CAD build for the part. Positions are in the model's coordinates, mm. A direction names the side the tool comes from. Coordinates: 2 decimals unless noted, no trailing zeros. Write each loop counter-clockwise with the first axis right and the second up, starting at its lowest first coordinate (ties: lowest second). Pieces come first, ordered by that corner, then holes. Notation, with made-up numbers: (14, -8) - (61, -8) arc R25 cw to (61, 20) - close; hole circle Ø5 at (12.5, 4.25). An arc over 180 degrees is marked (long way). One line per question, with ' | ' between items. Start each with the question number.
1. Two-plate mould, pull along X, no slides. Class faces 1 (the cylindrical face through (25.367, 8.972, -104.749)), 2 (the flat face through (-27, 7, -22)), 3 (the cylindrical face through (12.315, 5.423, -103.107)): +X half, -X half, draft (parallel to the pull), parting line (faces both ways), or undercut.
2. Which spindle directions (+Z, -Z, +X, -X, +Y, -Y) get a long thin tool onto all of the face, cutting with end or side? Do faces 4 (the cylindrical face through (-95.4, 2, -27.4)), 5 (the cylindrical face through (101.7, 2, -60.4)), 6 (the flat face through (1, 11, -63)), 7 (the cylindrical face through (-101.7, 2, -60.4)). Say none if no direction does.
3. Band-saw the part on A-A, the plane x = 65.5. Write the cut outline in (y, z), then the cut area to 3 significant figures.
4. Band-saw the part on B-B, the plane y = 4. Give the number of separate pieces and of enclosed holes in the cut face, then the cut area to 3 significant figures.
5. Flat gauge pins, fed straight in: P1, Ø1.5, axis at y = 2, z = -105.5, coming from the -X side; P2, Ø3, axis at x = -9.5, y = 15, coming from the -Z side. Where does each tip first touch, or does it go through?
6. Probe line 1 (X direction, y = 16, z = -30); line 2 (X direction, y = 16.75, z = -64); line 3 (X direction, y = 14.5, z = -64). List the from-to ranges inside material, lowest first.
from build123d import *

# Parameters (mm, degrees)
SKETCH2_W               = 195
SKETCH2_H               = 125
BOSS_EXTRUDE1_DEPTH     = 57
SKETCH3_W               = 181
SKETCH3_H               = 118
CUT_EXTRUDE1_DEPTH      = 50
BOSS_EXTRUDE2_DEPTH     = 15
CUT_EXTRUDE4_REACH      = 179.568
SKETCH7_R               = 2.75
SKETCH34_R              = 2
SKETCH34_W              = 22
SKETCH34_H              = 42
CUT_EXTRUDE8_DEPTH      = 7
MIRROR2_COPY_1_DEPTH    = 15
MIRROR2_COPY_2_REACH    = 179.568
MIRROR2_COPY_2_SKETCH_R = 2.75
MIRROR2_COPY_3_SKETCH_R = 2
MIRROR2_COPY_3_SKETCH_W = 22
MIRROR2_COPY_3_SKETCH_H = 42
MIRROR2_COPY_3_DEPTH    = 7
FILLET2_R               = 7
FILLET7_R               = 7
BOSS_EXTRUDE8_REACH     = 282.009
BOSS_EXTRUDE9_REACH     = 282.009
SKETCH29_W              = 460.325022979
SKETCH29_H              = 444.411594697
CUT_EXTRUDE5_DEPTH      = 50
SKETCH30_R              = 48
BOSS_EXTRUDE10_DEPTH    = 11
SKETCH31_R              = 41
CUT_EXTRUDE6_DEPTH      = 11
SKETCH32_R              = 3.2
CUT_EXTRUDE7_DEPTH      = 7
FILLET8_R               = 7
FILLET11_R              = 6.3
SKETCH37_W              = 42
SKETCH37_H              = 75
BOSS_EXTRUDE11_DEPTH    = 7
SKETCH39_W              = 259.645658498
SKETCH39_H              = 116.30884873
CUT_EXTRUDE9_DEPTH      = 125


with BuildPart() as part:
    # Sketch2 → Boss-Extrude1 (new body)
    with BuildSketch(Plane(origin=(0, 0, 0), x_dir=(1, 0, 0), z_dir=(0, 1, 0))):
        with Locations((0, -62.5)):
            Rectangle(SKETCH2_W, SKETCH2_H)
    boss_extrude1 = extrude(amount=BOSS_EXTRUDE1_DEPTH)

    # Sketch3 → Cut-Extrude1 (cut)
    with BuildSketch(Plane(origin=(0, 57, 0), x_dir=(1, 0, 0), z_dir=(0, 1, 0))):
        with Locations((0, -59)):
            Rectangle(SKETCH3_W, SKETCH3_H)
    cut_extrude1 = extrude(amount=-CUT_EXTRUDE1_DEPTH, mode=Mode.SUBTRACT)

    # Sketch5 → Boss-Extrude2 (add)
    with BuildSketch(Plane.ZY.offset(97.5)):
        Polygon((48.5, 7), (48.5, 0), (62.5, 0), (62.5, 57), (55.5, 57), (55.5, 7), align=None)
    boss_extrude2 = extrude(amount=BOSS_EXTRUDE2_DEPTH)

    # Sketch7 → Cut-Extrude4 (cut, up to next)
    with BuildSketch(Plane.XZ, mode=Mode.PRIVATE) as cut_extrude4_sk1:
        with Locations(Location((-82.5, 17.5, 0), (0, 0, 270))):
            Circle(SKETCH7_R)
    cut_extrude4_tool1 = extrude(cut_extrude4_sk1.sketch, amount=-CUT_EXTRUDE4_REACH, mode=Mode.PRIVATE) & part.part
    # Sketch7 → Cut-Extrude4 (cut, up to next)
    with BuildSketch(Plane.XZ, mode=Mode.PRIVATE) as cut_extrude4_sk2:
        with Locations(Location((-82.5, 110, 0), (0, 0, 270))):
            Circle(SKETCH7_R)
    cut_extrude4_tool2 = extrude(cut_extrude4_sk2.sketch, amount=-CUT_EXTRUDE4_REACH, mode=Mode.PRIVATE) & part.part
    cut_extrude4_1 = cut_extrude4_tool1.solids().sort_by_distance((-82.5, 0, 17.5))[0]
    add(cut_extrude4_1, mode=Mode.SUBTRACT)
    cut_extrude4_2 = cut_extrude4_tool2.solids().sort_by_distance((-82.5, 0, 110))[0]
    add(cut_extrude4_2, mode=Mode.SUBTRACT)
    cut_extrude4 = cut_extrude4_1 + cut_extrude4_2  # Cut-Extrude4 as one shape, for the pattern or mirror that repeats it

    # Sketch34 → Cut-Extrude8 (cut)
    with BuildSketch(Plane.XZ):
        with Locations(Location((-57.3, 88.85, 0), (0, 0, 270))):
            Circle(SKETCH34_R)
        with Locations(Location((-67.3, 88.85, 0), (0, 0, 270))):
            Circle(SKETCH34_R)
        with Locations(Location((-78.45, 63.75, 0), (0, 0, 270))):
            Circle(SKETCH34_R)
        with Locations(Location((-46.15, 63.75, 0), (0, 0, 270))):
            Circle(SKETCH34_R)
        with Locations(Location((-57.3, 38.65, 0), (0, 0, 270))):
            Circle(SKETCH34_R)
        with Locations(Location((-67.3, 38.65, 0), (0, 0, 270))):
            Circle(SKETCH34_R)
        with Locations((-62.3, 63.75)):
            Rectangle(SKETCH34_W, SKETCH34_H)
    cut_extrude8 = extrude(amount=-CUT_EXTRUDE8_DEPTH, mode=Mode.SUBTRACT)

    # Mirror1: Boss-Extrude2, Cut-Extrude4, Cut-Extrude8 across plane
    add(boss_extrude2.mirror(Plane(origin=(0, 0, 0), x_dir=(0, 0, 1), z_dir=(1, 0, 0))))
    add(cut_extrude4.mirror(Plane(origin=(0, 0, 0), x_dir=(0, 0, 1), z_dir=(1, 0, 0))), mode=Mode.SUBTRACT)
    add(cut_extrude8.mirror(Plane(origin=(0, 0, 0), x_dir=(0, 0, 1), z_dir=(1, 0, 0))), mode=Mode.SUBTRACT)

    # Mirror2: Boss-Extrude1, Cut-Extrude1, Boss-Extrude2, Cut-Extrude4, Cut-Extrude8 across plane
    add(boss_extrude1.mirror(Plane.XY))
    add(cut_extrude1.mirror(Plane.XY), mode=Mode.SUBTRACT)
    add(boss_extrude2.mirror(Plane.XY))
    add(cut_extrude4.mirror(Plane.XY), mode=Mode.SUBTRACT)
    add(cut_extrude8.mirror(Plane.XY), mode=Mode.SUBTRACT)

    # Mirror2 copy 1 sketch → Mirror2 copy 1 (add)
    with BuildSketch(Plane(origin=(97.5, 0, 0), x_dir=(0, 0, -1), z_dir=(1, 0, 0))):
        Polygon((48.5, 7), (48.5, 0), (62.5, 0), (62.5, 57), (55.5, 57), (55.5, 7), align=None)
    extrude(amount=MIRROR2_COPY_1_DEPTH)

    # Mirror2 copy 2 sketch → Mirror2 copy 2 (cut, up to next)
    with BuildSketch(Plane(origin=(0, 0, 0), x_dir=(-1, 0, 0), z_dir=(0, -1, 0)), mode=Mode.PRIVATE) as mirror2_copy_2_sk1:
        with Locations(Location((-82.5, 17.5, 0), (0, 0, 270))):
            Circle(MIRROR2_COPY_2_SKETCH_R)
    mirror2_copy_2_tool1 = extrude(mirror2_copy_2_sk1.sketch, amount=-MIRROR2_COPY_2_REACH, mode=Mode.PRIVATE) & part.part
    # Mirror2 copy 2 sketch → Mirror2 copy 2 (cut, up to next)
    with BuildSketch(Plane(origin=(0, 0, 0), x_dir=(-1, 0, 0), z_dir=(0, -1, 0)), mode=Mode.PRIVATE) as mirror2_copy_2_sk2:
        with Locations(Location((-82.5, 110, 0), (0, 0, 270))):
            Circle(MIRROR2_COPY_2_SKETCH_R)
    mirror2_copy_2_tool2 = extrude(mirror2_copy_2_sk2.sketch, amount=-MIRROR2_COPY_2_REACH, mode=Mode.PRIVATE) & part.part
    add(mirror2_copy_2_tool1.solids().sort_by_distance((82.5, 0, -17.5))[0], mode=Mode.SUBTRACT)
    add(mirror2_copy_2_tool2.solids().sort_by_distance((82.5, 0, -110))[0], mode=Mode.SUBTRACT)

    # Mirror2 copy 3 sketch → Mirror2 copy 3 (cut)
    with BuildSketch(Plane(origin=(0, 0, 0), x_dir=(-1, 0, 0), z_dir=(0, -1, 0))):
        with Locations(Location((-57.3, 88.85, 0), (0, 0, 270))):
            Circle(MIRROR2_COPY_3_SKETCH_R)
        with Locations(Location((-67.3, 88.85, 0), (0, 0, 270))):
            Circle(MIRROR2_COPY_3_SKETCH_R)
        with Locations(Location((-78.45, 63.75, 0), (0, 0, 270))):
            Circle(MIRROR2_COPY_3_SKETCH_R)
        with Locations(Location((-46.15, 63.75, 0), (0, 0, 270))):
            Circle(MIRROR2_COPY_3_SKETCH_R)
        with Locations(Location((-57.3, 38.65, 0), (0, 0, 270))):
            Circle(MIRROR2_COPY_3_SKETCH_R)
        with Locations(Location((-67.3, 38.65, 0), (0, 0, 270))):
            Circle(MIRROR2_COPY_3_SKETCH_R)
        with Locations((-62.3, 63.75)):
            Rectangle(MIRROR2_COPY_3_SKETCH_W, MIRROR2_COPY_3_SKETCH_H)
    extrude(amount=-MIRROR2_COPY_3_DEPTH, mode=Mode.SUBTRACT)

    # Fillet2
    fillet2_edges = [part.edges().sort_by_distance(p)[0] for p in [
        (-97.5, 28.5, -125),
        (97.5, 28.5, -125),
        (97.5, 28.5, 125),
        (-97.5, 28.5, 125),
    ]]
    fillet(fillet2_edges, radius=FILLET2_R)

    # Fillet7
    fillet7_edges = [part.edges().sort_by_distance(p)[0] for p in [
        (97.5, 0, 0),
        (-97.5, 0, 0),
        (97.5, 0, -90.25),
        (-97.5, 0, 90.25),
        (97.5, 0, 90.25),
        (-97.5, 0, -90.25),
        (0, 0, -125),
        (0, 0, 125),
        (112.5, 0, 55.5),
        (105, 0, 62.5),
        (105, 0, 48.5),
        (-112.5, 0, -55.5),
        (-105, 0, -62.5),
        (-105, 0, -48.5),
        (105, 0, -48.5),
        (105, 0, -62.5),
        (112.5, 0, -55.5),
        (-105, 0, 48.5),
        (-105, 0, 62.5),
        (-95.449747468, 0, 122.949747468),
        (-95.449747468, 0, -122.949747468),
        (95.449747468, 0, -122.949747468),
        (95.449747468, 0, 122.949747468),
        (-112.5, 0, 55.5),
    ]]
    fillet(fillet7_edges, radius=FILLET7_R - 0.0001)  # a hair under: the kernel refuses the full size

    # Sketch26 → Boss-Extrude8 (add, up to next)
    with BuildSketch(Plane.XY.offset(125), mode=Mode.PRIVATE) as boss_extrude8_sk1:
        with BuildLine():
            Line((-90.5, 7), (90.5, 7))
            ThreePointArc((90.5, 7), (88.449747468, 2.050252532), (83.5, 0))
            Line((83.5, 0), (-83.5, 0))
            ThreePointArc((-83.5, 0), (-88.449747468, 2.050252532), (-90.5, 7))
        make_face()
    boss_extrude8_tool1 = extrude(boss_extrude8_sk1.sketch, amount=-BOSS_EXTRUDE8_REACH, mode=Mode.PRIVATE) - part.part
    add(boss_extrude8_tool1.solids().sort_by_distance((0, 3.532685, 125))[0])

    # Sketch27 → Boss-Extrude9 (add, up to next)
    with BuildSketch(Plane(origin=(0, 0, -125), x_dir=(-1, 0, 0), z_dir=(0, 0, -1)), mode=Mode.PRIVATE) as boss_extrude9_sk1:
        with BuildLine():
            Line((-90.5, 7), (90.5, 7))
            ThreePointArc((90.5, 7), (88.449747468, 2.050252532), (83.5, 0))
            Line((83.5, 0), (-83.5, 0))
            ThreePointArc((-83.5, 0), (-88.449747468, 2.050252532), (-90.5, 7))
        make_face()
    boss_extrude9_tool1 = extrude(boss_extrude9_sk1.sketch, amount=-BOSS_EXTRUDE9_REACH, mode=Mode.PRIVATE) - part.part
    add(boss_extrude9_tool1.solids().sort_by_distance((0, 3.532685, -125))[0])

    # Sketch29 → Cut-Extrude5 (cut)
    with BuildSketch(Plane(origin=(0, 57, 0), x_dir=(1, 0, 0), z_dir=(0, 1, 0))):
        with Locations((1.552529588, 6.210118353)):
            Rectangle(SKETCH29_W, SKETCH29_H)
    extrude(amount=-CUT_EXTRUDE5_DEPTH, mode=Mode.SUBTRACT)

    # Sketch30 → Boss-Extrude10 (add)
    with BuildSketch(Plane(origin=(0, 7, 0), x_dir=(1, 0, 0), z_dir=(0, 1, 0))):
        with Locations(Location((0, 64, 0), (0, 0, 0.616739929))):
            Circle(SKETCH30_R)
    extrude(amount=BOSS_EXTRUDE10_DEPTH)

    # Sketch31 → Cut-Extrude6 (cut)
    with BuildSketch(Plane.XZ):
        with Locations(Location((0, -64, 0), (0, 0, 270))):
            Circle(SKETCH31_R)
    extrude(amount=-CUT_EXTRUDE6_DEPTH, mode=Mode.SUBTRACT)

    # Sketch32 → Cut-Extrude7 (cut)
    with BuildSketch(Plane.XZ.offset(-11)):
        with Locations(Location((0, -30, 0), (0, 0, 270))):
            Circle(SKETCH32_R)
        with Locations(Location((0, -98, 0), (0, 0, 270))):
            Circle(SKETCH32_R)
        with Locations(Location((34, -64, 0), (0, 0, 270))):
            Circle(SKETCH32_R)
        with Locations(Location((-34, -64, 0), (0, 0, 270))):
            Circle(SKETCH32_R)
    extrude(amount=-CUT_EXTRUDE7_DEPTH, mode=Mode.SUBTRACT)

    # Fillet8
    fillet8_edges = [part.edges().sort_by_distance(p)[0] for p in [
        (-47.997219225, 18, -63.483331143),
    ]]
    fillet(fillet8_edges, radius=FILLET8_R)

    # Fillet11
    fillet11_edges = [part.edges().sort_by_distance(p)[0] for p in [
        (73.3, 3.5, 84.75),
        (73.3, 3.5, 42.75),
        (51.3, 3.5, 42.75),
        (51.3, 3.5, 84.75),
        (-51.3, 3.5, 42.75),
        (-51.3, 3.5, 84.75),
        (-73.3, 3.5, 84.75),
        (-73.3, 3.5, 42.75),
    ]]
    fillet(fillet11_edges, radius=FILLET11_R)

    # Sketch37 → Boss-Extrude11 (add)
    with BuildSketch(Plane.XZ):
        with Locations((64.5, -62.5)):
            Rectangle(SKETCH37_W, SKETCH37_H)
        with Locations((-64.5, -62.5)):
            Rectangle(SKETCH37_W, SKETCH37_H)
    extrude(amount=-BOSS_EXTRUDE11_DEPTH)

    # Sketch39 → Cut-Extrude9 (cut)
    with BuildSketch(Plane.XY.offset(125)):
        with Locations((-5.095435278, 8.271148339)):
            Rectangle(SKETCH39_W, SKETCH39_H)
    extrude(amount=-CUT_EXTRUDE9_DEPTH, mode=Mode.SUBTRACT)


solid = part.part
Filled in:
1) face 1: parting line | face 2: draft | face 3: undercut
2) face 4: +Z, -X, -Y | face 5: -Z, +X, -Y | face 6: -Y | face 7: -Z, -X, -Y
3) outline: (0, -125) - (7, -125) - (7, 0) - (0, 0) - close | area: 875 mm²
4) separate pieces: 1 | enclosed holes: 5 | area: 19,200 mm²
5) P1: stops at x = -96.06 | P2: stops at z = -110.65
6) line 1: x = -30.83 to -3.2, 3.2 to 30.83 | line 2: x = -44.99 to -37.2, -30.8 to 30.8, 37.2 to 44.99 | line 3: x = -47.06 to -37.2, -30.8 to 30.8, 37.2 to 47.06
